from build123d import *

# Parameters (mm, degrees)
F0_W     = 25.4
F0_H     = 57.15
F1_DEPTH = 44.45
F2_W     = 44.45
F2_H     = 31.75
F3_DEPTH = 25.4
F5_DEPTH = 25.4
F7_DEPTH = 25.4
F8_R     = 6.35
F9_DEPTH = 25.4


with BuildPart() as f1:
    # F0 (on Top) → F1 (new body)
    with BuildSketch(Plane.XY):
        with Locations((12.7, 28.575)):
            Rectangle(F0_W, F0_H)
    extrude(amount=F1_DEPTH)

    # F2 (on face) → F3 (cut)
    with BuildSketch(Plane(origin=(0, 0, 0), x_dir=(0, -1, 0), z_dir=(-1, 0, 0))):
        with Locations((-22.225, 28.575)):
            Rectangle(F2_W, F2_H)
    extrude(amount=-F3_DEPTH, mode=Mode.SUBTRACT)

    # F4 (on face) → F5 (cut)
    with BuildSketch(Plane(origin=(0, 57.15, 0), x_dir=(-1, 0, 0), z_dir=(0, 1, 0))):
        with BuildLine():
            ThreePointArc((-25.4, 31.75), (-21.6802561211, 40.7302561211), (-12.7, 44.45))
            Line((-12.7, 44.45), (-25.4, 44.45))
            Line((-25.4, 44.45), (-25.4, 31.75))
        make_face()
        with BuildLine():
            ThreePointArc((-12.7, 44.45), (-3.7197438789, 40.7302561211), (0, 31.75))
            Line((0, 31.75), (0, 44.45))
            Line((0, 44.45), (-12.7, 44.45))
        make_face()
    extrude(amount=-F5_DEPTH, mode=Mode.SUBTRACT)

    # F6 (on face) → F7 (cut)
    with BuildSketch(Plane(origin=(0, 57.15, 0), x_dir=(-1, 0, 0), z_dir=(0, 1, 0))):
        with BuildLine():
            add(Edge.make_bspline(
                [(-6.35, 31.75), (-6.35, 38.1), (-12.7, 38.1), (-19.05, 38.1), (-19.05, 31.75)],
                knots=[0, 0, 0, 1.5707963268, 1.5707963268, 3.1415926536, 3.1415926536, 3.1415926536], degree=2, weights=[1, 0.7071067812, 1, 0.7071067812, 1]))
            Line((-6.35, 31.75), (-6.35, 42.7485226281))
            ThreePointArc((-6.35, 42.7485226281), (-12.7, 44.45), (-19.05, 42.7485226281))
            Line((-19.05, 42.7485226281), (-19.05, 31.75))
        make_face()
        with BuildLine():
            add(Edge.make_bspline(
                [(-19.05, 31.75), (-19.05, 25.4), (-12.7, 25.4), (-6.35, 25.4), (-6.35, 31.75)],
                knots=[3.1415926536, 3.1415926536, 3.1415926536, 4.7123889804, 4.7123889804, 6.2831853072, 6.2831853072, 6.2831853072], degree=2, weights=[1, 0.7071067812, 1, 0.7071067812, 1]))
            add(Edge.make_bspline(
                [(-6.35, 31.75), (-6.35, 38.1), (-12.7, 38.1), (-19.05, 38.1), (-19.05, 31.75)],
                knots=[0, 0, 0, 1.5707963268, 1.5707963268, 3.1415926536, 3.1415926536, 3.1415926536], degree=2, weights=[1, 0.7071067812, 1, 0.7071067812, 1]))
        make_face()
    extrude(amount=-F7_DEPTH, mode=Mode.SUBTRACT)

    # F8 (on face) → F9 (cut)
    with BuildSketch(Plane.XY.offset(12.7)):
        with Locations((12.7, 31.75)):
            Circle(F8_R)
        with Locations((12.7, 12.7)):
            Circle(F8_R)
    extrude(amount=-F9_DEPTH, mode=Mode.SUBTRACT)


solid = f1.part
Could you check a few things on this model? Use its own coordinates, in mm. A direction names the side the tool comes from. Coordinates: 2 decimals unless noted, no trailing zeros. Order: outer loops, then holes, each group sorted by start corner. A loop starts at its lowest first (then second) coordinate and runs counter-clockwise, first axis right, second up. Notation, with made-up numbers: (-34.75, 16.25) -> (3.25, 16.25) arc R19 ccw to (3.25, 29.25) -> close; hole circle Ø6 at (77.5, -15.5). An arc over 180 degrees is marked (long way). One line per item, written item: value. Start each with the question number.
1) If I drill on L1, parallel to Y at x = 12.7, z = 9; L2, parallel to Z at x = 7, y = 26; L3, parallel to X at y = 31, z = 9, over which ranges is the centre line in solid material (lowest first)? Write a range as [from, to].
2) We'd pull the mould along Y, two halves only. Please class faces 1 (the flat face through (13, 44.45, 24)), 2 (the flat face through (0, 35, 9)), 3 (the cylindrical face through (8.02, 16.99, 6.44)): +Y half, -Y half, draft (parallel to the pull), parting line (faces both ways), or undercut.
3) Imagine slicing it at B-B on z = 5. List the corners of the cut face in (x, y) for me, plus the area to 3 significant figures.
4) I'm going to push flat-ended pins straight in: pin 1 (5.5 mm diameter, centred on y = 50, z = 38.5, fed in from -X); pin 2 (4 mm diameter, centred on x = 18, y = 15, fed in from +Z); pin 3 (1 mm diameter, centred on x = 17, z = 22, fed in from -Y). Where does each tip first touch, or does it pass through?
5) Which directions (+Z, -Z, +X, -X, +Y, -Y) give clear straight access to the entire face, cutting with the end or side of a thin tool? Please do faces 4 (the flat face through (13, 23, 12.7)), 5 (the flat face through (6.35, 51, 37)), 6 (the flat face through (13, 0, 6)).
6) Imagine slicing it at A-A on y = 12.7. List the corners of the cut face in (x, z) for me, plus the area to 3 significant figures.
7) Imagine slicing it at C-C on x = 12.7. Count the separate pieces of the cut face and the enclosed holes in it, plus the area to 3 significant figures.
8) Imagine slicing it at D-D on y = 36. List the corners of the cut face in (x, z) for me, plus the area to 3 significant figures.
Answer list:
1. L1: y = [0, 6.35], [19.05, 25.4], [38.1, 57.15]
1. L2: z = [0, 12.7]
1. L3: x = [0, 6.39], [19.01, 25.4]
2. face 1: -Y half
2. face 2: draft
2. face 3: undercut
3. outline: (0, 0) -> (25.4, 0) -> (25.4, 57.15) -> (0, 57.15) -> close; hole circle Ø12.7 at (12.7, 12.7); hole circle Ø12.7 at (12.7, 31.75)
3. area: 1,200 mm2
4. pin 1: stops at x = 0.65
4. pin 2: stops at z = 12.7
4. pin 3: stops at y = 44.45
5. face 4: +Z, +X, -X, -Y
5. face 5: +Z, +Y, -Y
5. face 6: +Z, -Z, +X, -X, -Y
6. outline: (0, 0) -> (6.35, 0) -> (6.35, 12.7) -> (0, 12.7) -> close; (19.05, 0) -> (25.4, 0) -> (25.4, 12.7) -> (19.05, 12.7) -> close
6. area: 161 mm2
7. separate pieces: 3
7. enclosed holes: 0
7. area: 565 mm2
8. outline: (0, 0) -> (7.98, 0) -> (7.98, 12.7) -> (0, 12.7) -> close; (17.42, 0) -> (25.4, 0) -> (25.4, 12.7) -> (17.42, 12.7) -> close
8. area: 203 mm2
